For this review, take the finished solid that the model builds, in its own axes (mm). Face numbers are marked on the shaded views. A direction names the side the tool comes from. Round coordinates to 2 decimals unless told otherwise and drop trailing zeros. Write each loop counter-clockwise with the first axis right and the second up, starting at its lowest first coordinate (ties: lowest second). Pieces come first, ordered by that corner, then holes.
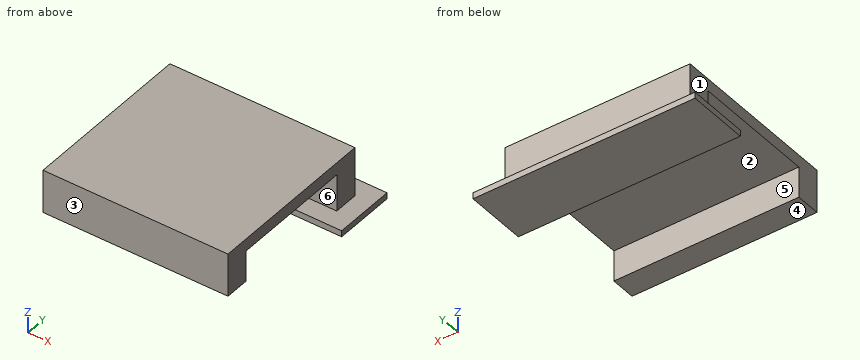
from build123d import *

# Parameters (mm, degrees)
SKETCH1_W           = 38.1
SKETCH1_H           = 5.08
BOSS_EXTRUDE1_DEPTH = 2.54
SKETCH2_W           = 38.1
SKETCH2_H           = 2.54
BOSS_EXTRUDE2_DEPTH = 30.48
SKETCH3_W           = 38.1
SKETCH3_H           = 5.08
BOSS_EXTRUDE3_DEPTH = 7.62
SKETCH4_W           = 38.1
SKETCH4_H           = 5.08
BOSS_EXTRUDE4_DEPTH = 6.35
SKETCH5_W           = 45.72
SKETCH5_H           = 12.7
BOSS_EXTRUDE5_DEPTH = 1.27


with BuildPart() as part:
    # Sketch1 → Boss-Extrude1 (new body)
    with BuildSketch(Plane.XY):
        Rectangle(SKETCH1_W, SKETCH1_H)
    extrude(amount=BOSS_EXTRUDE1_DEPTH)

    # Sketch2 → Boss-Extrude2 (add)
    with BuildSketch(Plane(origin=(0, 2.54, 0), x_dir=(1, 0, 0), z_dir=(0, 1, 0))):
        with Locations((0, -1.27)):
            Rectangle(SKETCH2_W, SKETCH2_H)
    extrude(amount=BOSS_EXTRUDE2_DEPTH)

    # Sketch3 → Boss-Extrude3 (add)
    with BuildSketch(Plane(origin=(0, 0, 0), x_dir=(-1, 0, 0), z_dir=(0, 0, -1))):
        with Locations((0, 30.48)):
            Rectangle(SKETCH3_W, SKETCH3_H)
    extrude(amount=BOSS_EXTRUDE3_DEPTH)

    # Sketch4 → Boss-Extrude4 (add)
    with BuildSketch(Plane(origin=(0, 0, 0), x_dir=(-1, 0, 0), z_dir=(0, 0, -1))):
        Rectangle(SKETCH4_W, SKETCH4_H)
    extrude(amount=BOSS_EXTRUDE4_DEPTH)

    # Sketch5 → Boss-Extrude5 (add)
    with BuildSketch(Plane(origin=(0, 0, -7.62), x_dir=(-1, 0, 0), z_dir=(0, 0, -1))):
        with Locations((0, 30.48)):
            Rectangle(SKETCH5_W, SKETCH5_H)
    extrude(amount=BOSS_EXTRUDE5_DEPTH)


solid = part.part
(1) We need section B-B, the plane x = 8. Give the boundary of the cut face in (y, z).
Geometry check:
outline: (-2.54, -6.35) - (2.54, -6.35) - (2.54, 0) - (27.94, 0) - (27.94, -7.62) - (24.13, -7.62) - (24.13, -8.89) - (36.83, -8.89) - (36.83, -7.62) - (33.02, -7.62) - (33.02, 2.54) - (-2.54, 2.54) - close
(2) For line 1 along Y through (x, z) = (9, -1); line 2 along Z through (x, y) = (-4.5, 25.5); line 3 along Z through (x, y) = (2.5, 21.5), list the stretches that pass through material, from the lowest coordinate up.
Geometry check:
line 1: y = -2.54 to 2.54, 27.94 to 33.02
line 2: z = -8.89 to -7.62, 0 to 2.54
line 3: z = 0 to 2.54
(3) For the marked faces 4, 5 and 6, list the 3-axis set-ups (+Z, -Z, +X, -X, +Y, -Y) from which the entire face can be reached by the end or side of a thin tool; tool diameter is ignored.
Geometry check:
face 4: -Z, +X, -X, -Y
face 5: -Z, +X, -X
face 6: +X, -X
(4) For pin 1 Ø4 at (x, y) = (6.5, 1) entering from -Z; pin 2 Ø1 at (x, y) = (-6, 9) entering from -Z; pin 3 Ø1 at (x, z) = (16, -2) entering from +Y, all flat-tipped, find the tip position at first contact; note any pin that passes through.
Geometry check:
pin 1: stops at z = -6.35
pin 2: stops at z = 0
pin 3: stops at y = 33.02
(5) We need section D-D, the plane z = 0.5. Give the boundary of the cut face in (x, y).
Geometry check:
outline: (-19.05, -2.54) - (19.05, -2.54) - (19.05, 33.02) - (-19.05, 33.02) - close
(6) We need section C-C, the plane y = 30. Give the boundary of the cut face in (x, z).
Geometry check:
outline: (-22.86, -8.89) - (22.86, -8.89) - (22.86, -7.62) - (19.05, -7.62) - (19.05, 2.54) - (-19.05, 2.54) - (-19.05, -7.62) - (-22.86, -7.62) - close
(7) Mouldability with a two-part tool opening along Y and no side actions: class the marked faces 1, 2 and 3 as pulls with the +Y half, pulls with the -Y half, needs draft (parallel to the pull), parting line crosses it, or undercut.
Geometry check:
face 1: needs draft
face 2: undercut
face 3: pulls with the -Y half
(8) We need section A-A, the plane z = -4.75. Give the boundary of the cut face in (x, y).
Geometry check:
outline: (-19.05, -2.54) - (19.05, -2.54) - (19.05, 2.54) - (-19.05, 2.54) - close; (-19.05, 27.94) - (19.05, 27.94) - (19.05, 33.02) - (-19.05, 33.02) - close
